Part model, mm, in its own coordinate system. Round coordinates to 2 decimals unless told otherwise and drop trailing zeros. Loops run counter-clockwise (first coordinate to the right, second up) from the corner with the lowest first, then second, coordinate; pieces in that order, holes last.
(1) Cut at C-C on z = -41. List the corners of the cut face in (x, y), then the cut area to 3 significant figures.
(2) Cut at A-A on z = 6.5. List the corners of the cut face in (x, y).
(3) Cut at D-D on y = 4.1. Count the separate pieces of the cut face and the enclosed holes in it, then the cut area to 3 significant figures.
(4) Flat gauge pins, fed straight in: pin 1 (4.5 mm diameter, centred on x = -41, z = -41, fed in from -Y); pin 2 (2 mm diameter, centred on y = 2.5, z = 49, fed in from +X); pin 3 (2 mm diameter, centred on y = 3, z = -26.5, fed in from +X); pin 4 (3.5 mm diameter, centred on x = -17.28, z = -2.76, fed in from -Y). Where does each tip first touch, or does it go through?
(5) Cut at B-B on x = 41. List the corners of the cut face in (y, z).
(6) Mould opens along X. For faces 1 (the face through (-43, 3, -41)), 2 (the face through (1, 0, 14)), 3 (the face through (-5.037, 2.535, 12.147)), 4 (the face through (19.52, 2.46, 62)) say: +X half, -X half, draft (parallel to the pull), parting line (faces both ways), or undercut.
(7) Probe probe 1 along X at (y, z) = (2.15, 41); probe 2 along X at (y, z) = (3, 40); probe 3 along Z at (x, y) = (-5.5, 3.85). List the from-to ranges inside material, lowest first.
from build123d import *

# Parameters (mm, degrees)
SKETCH1_R           = 65
BOSS_EXTRUDE1_DEPTH = 5
SKETCH2_R           = 13.15
SKETCH2_R_2         = 2
CUT_EXTRUDE1_DEPTH  = 93.059763198
SKETCH4_R           = 2
CUT_EXTRUDE2_DEPTH  = 93.059763198


with BuildPart() as part:
    # Sketch1 → Boss-Extrude1 (new body)
    with BuildSketch(Plane(origin=(0, 0, 0), x_dir=(1, 0, 0), z_dir=(0, 1, 0))):
        with Locations(Location((0, 0, 0), (0, 0, 270))):
            Circle(SKETCH1_R)
    extrude(amount=BOSS_EXTRUDE1_DEPTH)

    # Sketch2 → Cut-Extrude1 (cut, through all)
    with BuildSketch(Plane(origin=(0, 5, 0), x_dir=(1, 0, 0), z_dir=(0, 1, 0))):
        with Locations(Location((0, 0, 0), (0, 0, 270))):
            Circle(SKETCH2_R)
        with Locations(Location((-17.281297977, 2.75803195, 0), (0, 0, 270))):
            Circle(SKETCH2_R_2)
        with Locations(Location((2.75803195, 17.281297977, 0), (0, 0, 270))):
            Circle(SKETCH2_R_2)
        with Locations(Location((17.281297977, -2.75803195, 0), (0, 0, 270))):
            Circle(SKETCH2_R_2)
        with Locations(Location((-2.75803195, -17.281297977, 0), (0, 0, 270))):
            Circle(SKETCH2_R_2)
    extrude(amount=-CUT_EXTRUDE1_DEPTH, mode=Mode.SUBTRACT)

    # Sketch4 → Cut-Extrude2 (cut, through all)
    with BuildSketch(Plane(origin=(0, 5, 0), x_dir=(1, 0, 0), z_dir=(0, 1, 0))):
        with Locations(Location((41, 41, 0), (0, 0, 270))):
            Circle(SKETCH4_R)
        with Locations(Location((41, -41, 0), (0, 0, 270))):
            Circle(SKETCH4_R)
        with Locations(Location((-41, -41, 0), (0, 0, 270))):
            Circle(SKETCH4_R)
        with Locations(Location((-41, 41, 0), (0, 0, 270))):
            Circle(SKETCH4_R)
    extrude(amount=-CUT_EXTRUDE2_DEPTH, mode=Mode.SUBTRACT)


solid = part.part
Final values:
1. outline: (-50.44, 0) - (-43, 0) - (-43, 5) - (-50.44, 5) - close; (-39, 0) - (39, 0) - (39, 5) - (-39, 5) - close; (43, 0) - (50.44, 0) - (50.44, 5) - (43, 5) - close
1. area: 464 mm2
2. outline: (-64.67, 0) - (-11.43, 0) - (-11.43, 5) - (-64.67, 5) - close; (11.43, 0) - (64.67, 0) - (64.67, 5) - (11.43, 5) - close
3. separate pieces: 1
3. enclosed holes: 9
3. area: 12,600 mm2
4. pin 1: stops at y = 0
4. pin 2: stops at x = 43.83
4. pin 3: stops at x = 59.79
4. pin 4: passes through
5. outline: (0, -50.44) - (5, -50.44) - (5, -43) - (0, -43) - close; (0, -39) - (5, -39) - (5, 39) - (0, 39) - close; (0, 43) - (5, 43) - (5, 50.44) - (0, 50.44) - close
6. face 1: undercut
6. face 2: draft
6. face 3: undercut
6. face 4: parting line
7. probe 1: x = -50.44 to -43, -39 to 39, 43 to 50.44
7. probe 2: x = -51.23 to -42.73, -39.27 to 39.27, 42.73 to 51.23
7. probe 3: z = -64.77 to -11.94, 11.94 to 64.77
